Autodesk Inventor part; units mm, degrees
ref_plane "YZ Plane" through (0, 0, 0) normal (1, 0, 0) x (0, 1, 0)
ref_plane "XZ Plane" through (0, 0, 0) normal (0, 1, 0) x (-1, 0, 0)
ref_plane "XY Plane" through (0, 0, 0) normal (0, 0, 1) x (1, 0, 0)
sketch "Sketch1" plane through (0, 0, 0) normal (0, 0, 1) x (1, 0, 0)
  line L0 (0, 0) -> (30, 0)
  line L1 (30, 0) -> (30, 200)
  line L2 (30, 200) -> (0, 200)
  line L3 (0, 200) -> (0, 0)
  dimension "d0" = 30
  dimension "d1" = 200
extrude "Extrusion1" add sketch "Sketch1" along normal blind 40
sketch "Sketch2" plane through (0, 0, 0) normal (-1, 0, 0) x (0, 0, 1)
  line L0 (0, 0) -> (33, 0)
  line L1 (33, 0) -> (33, 33.5)
  line L2 (33, 33.5) -> (0, 33.5)
  line L3 (0, 33.5) -> (0, 0)
  dimension "d4" = 33
  dimension "d5" = 33.5
extrude "Extrusion2" cut sketch "Sketch2" against normal up to surface (30 mm away)
sketch "Sketch3" plane through (0, 0, 33) normal (0, 0, -1) x (-1, 0, 0)
  circle A0 centre (-15, 18) radius 3.95
  line L0 (0, 0) -> (-30, 0)
  line L1 (0, 33.5) -> (0, 0)
  dimension "d8" = 7.9
  dimension "d9" = 18
  dimension "d10" = 15
extrude "Extrusion3" add sketch "Sketch3" along normal blind 7
sketch "Sketch5" plane through (0, 0, 40) normal (0, 0, 1) x (1, 0, 0)
  line L0 (0, 33.5) -> (0, 0)
  line L1 (30, 0) -> (30, 200)
  line L2 (0, 0) -> (30, 0)
  line L3 (30, 0) -> (30, 10)
  line L4 (30, 10) -> (0, 10)
  line L5 (0, 10) -> (0, 0)
  dimension "d16" = 10
extrude "Extrusion5" cut sketch "Sketch5" against normal up to surface (7 mm away)
sketch "Sketch7" plane through (0, 0, 40) normal (0, 0, 1) x (1, 0, 0)
  circle A0 centre (15, 185) radius 4
  line L0 (30, 200) -> (0, 200)
  line L1 (30, 10) -> (30, 200)
  point P0 (0, 0)
  dimension "d19" = 8
  dimension "d22" = 15
  dimension "d23" = 15
extrude "Extrusion6" add sketch "Sketch7" along normal blind 7
sketch "Sketch8" plane through (0, 33.5, 0) normal (0, -1, 0) x (1, 0, 0)
  line L0 (30, 33) -> (30, 0)
  line L1 (0, 33) -> (30, 33)
  line L2 (0, 0) -> (0, 33)
  line L3 (30, 0) -> (0, 0)
  line L4 (3, 30) -> (27, 30)
  line L5 (27, 30) -> (27, 3)
  line L6 (27, 3) -> (3, 3)
  line L7 (3, 3) -> (3, 30)
  point P0 (0, 0)
  dimension "d24" = 3
extrude "Extrusion7" cut sketch "Sketch8" against normal up to surface (166.5 mm away) contours L4 L5 L6 L7
sketch "Sketch9" plane through (0, 0, 40) normal (0, 0, 1) x (1, 0, 0)
  circle A0 centre (15, 18) radius 3.95
  line L0 (0, 200) -> (0, 10)
  line L1 (30, 10) -> (30, 33.5)
  arc A1 (0, 18) -> (30, 18) centre (15, 28.0625) ccw
  line L2 (30, 10) -> (0, 10)
  line L3 (0, 18) -> (0, 10)
  line L4 (0, 10) -> (30, 10)
  line L5 (30, 18) -> (30, 10)
  line L6 (15, 18) -> (15, 28.0625) construction
  point P0 (0, 0)
  point P1 (15, 10)
  dimension "d27" = 8
extrude "Extrusion8" cut sketch "Sketch9" against normal up to surface (7 mm away) contours A1 L2 L0 | A1 L1 L2
properties part number "arm1"
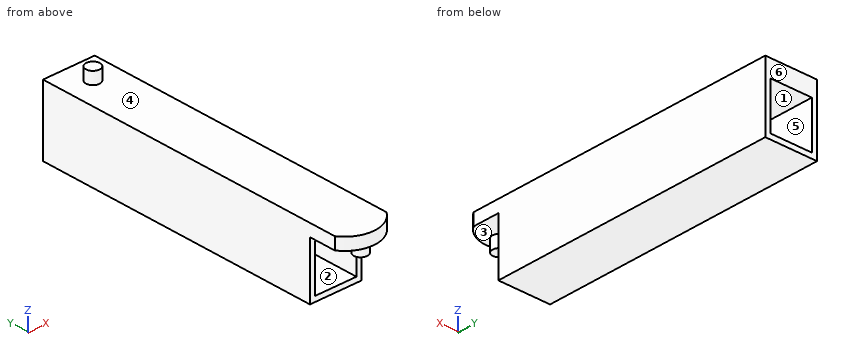
Verification items for the finished model (mm, model axes). Face numbers are marked on the shaded views. A direction names the side the tool comes from. Give positions to 0.01 mm unless a question says otherwise; leave off trailing zeros. Loops run counter-clockwise (first coordinate to the right, second up) from the corner with the lowest first, then second, coordinate; pieces in that order, holes last. Notation, with made-up numbers: M 18,-33 L 55,-33 A25 cw 55,-1 Z; hole C 84,20 d8. An arc over 180 degrees is marked long. Return JSON: item names as keys, results as strings.
1) Tool access check on the marked faces 5 and 6. Record the directions out of +Z, -Z, +X, -X, +Y, -Y that give a thin tool (end or side, any length) a straight path to the whole face; none if there is none.
Findings:
{"face 5": "+Y, -Y", "face 6": "+Z, -Z, +X, -X, +Y"}
2) Gauge pin test, flat ends, axial feed: P1, Ø12, axis at x = 11, y = 86.5, coming from the +Z side; P2, Ø15, axis at x = 14, z = 19, coming from the -Y side; P3, Ø8.5, axis at x = 16, y = 16.5, coming from the -Z side. Record the tip position at first contact, or that the pin passes through.
Findings:
{"P1": "stops at z = 40", "P2": "stops at y = 14.05", "P3": "stops at z = 26"}
3) Mould release check, pull along Z, two halves, no side actions. Record for the marked faces 1, 2, 3 and 4: released by +Z, released by -Z, zero draft, split by the parting line, or undercut.
Findings:
{"face 1": "undercut", "face 2": "undercut", "face 3": "released by -Z", "face 4": "released by +Z"}
4) Section check C-C, the plane y = 141. Enter the section's corners in (x, z).
Findings:
{"outline": "M 0,0 L 30,0 L 30,40 L 0,40 Z; hole M 3,3 L 27,3 L 27,30 L 3,30 Z"}
5) Material ranges on L1, parallel to X at y = 109, z = 16.5; L2, parallel to Z at x = 21, y = 97; L3, parallel to Z at x = 27.25, y = 175.5, recorded low to high. Write a range as [from, to].
Findings:
{"L1": "x = [0, 3], [27, 30]", "L2": "z = [0, 3], [30, 40]", "L3": "z = [0, 40]"}
6) Section check D-D, the plane y = 185. Enter the section's corners in (x, z), and give its area (3 significant figures).
Findings:
{"outline": "M 0,0 L 30,0 L 30,40 L 19,40 L 19,47 L 11,47 L 11,40 L 0,40 Z; hole M 3,3 L 27,3 L 27,30 L 3,30 Z", "area": "608 mm2"}
7) Section check A-A, the plane x = 15. Enter the section's corners in (y, z), and give its area (3 significant figures).
Findings:
{"outline": "M 10,33 L 14.05,33 L 14.05,26 L 21.95,26 L 21.95,33 L 33.5,33 L 33.5,30 L 200,30 L 200,40 L 189,40 L 189,47 L 181,47 L 181,40 L 10,40 Z; M 33.5,0 L 200,0 L 200,3 L 33.5,3 Z", "area": "2,440 mm2"}
8) Section check B-B, the plane z = 24. Enter the section's corners in (x, y).
Findings:
{"outline": "M 0,33.5 L 3,33.5 L 3,200 L 0,200 Z; M 27,33.5 L 30,33.5 L 30,200 L 27,200 Z"}
